```python
from build123d import *

# Parameters (mm, degrees)
SKETCH_1_R      = 2.1
EXTRUDE_1_DEPTH = 3


with BuildPart() as part:
    # 스케치1 → 보스-돌출1 (new, symmetric)
    with BuildSketch(Plane.XY):
        with BuildLine():
            Line((-4.654662174, -7.079831659), (-4.654662174, 5.301751688))
            Line((-4.654662174, 5.301751688), (10.655145319, 5.301751688))
            ThreePointArc((10.655145319, 5.301751688), (12.164725545, 4.600439307), (13.28874021, 3.372733093))
            Line((13.28874021, 3.372733093), (13.28874021, 2.168909846))
            ThreePointArc((13.28874021, 2.168909846), (11.333538367, 0.764001831), (8.927874518, 0.66724324))
            Line((8.927874518, 0.66724324), (3.345337826, 0.66724324))
            Line((3.345337826, 0.66724324), (3.345337826, -6.968753808))
            ThreePointArc((3.345337826, -6.968753808), (0.343177667, -8.564508011), (-0.439769501, -11.873041045))
            ThreePointArc((-0.439769501, -11.873041045), (-1.484211123, -14.014409685), (-3.830025316, -13.597907913))
            ThreePointArc((-3.830025316, -13.597907913), (-5.564151963, -10.506098848), (-4.654662174, -7.079831659))
        make_face()
        Circle(SKETCH_1_R, mode=Mode.SUBTRACT)
    extrude(amount=EXTRUDE_1_DEPTH, both=True)


solid = part.part
```
CAD build for the part. Positions are in the model's coordinates, mm. A direction names the side the tool comes from. Round coordinates to 2 decimals unless told otherwise and drop trailing zeros. Loops run counter-clockwise (first coordinate to the right, second up) from the corner with the lowest first, then second, coordinate; pieces in that order, holes last. Notation, with made-up numbers: M 9,21.5 L 36,21.5 A25 ccw 36,47.5 Z; hole C 33.5,26 d4. An arc over 180 degrees is marked long. Return JSON: item names as keys, results as strings. Group by question number.
(1) Tool access for faces 1 (the flat face through (3, 5.302, 0)), 2 (the flat face through (-4.655, -1, 0)), 3 (the flat face through (6, 0.667, 0)): list every direction of +Z, -Z, +X, -X, +Y, -Y with a clear straight run to the whole face (end or side of a thin tool).
(2) Saw through at C-C, the plane z = 0. List the corners of the cut face in (x, y), and give its area (3 significant figures).
(3) Saw through at B-B, the plane y = 0. List the corners of the cut face in (x, z).
(4) Saw through at A-A, the plane x = 0. List the corners of the cut face in (y, z).
(5) Mould opens along Y. For faces 4 (the cylindrical face through (12.15, 4.61, 0.04)), 5 (the cylindrical face through (0.37, -8.53, 0.04)), 6 (the flat face through (13.289, 3, 0)) say: +Y half, -Y half, draft (parallel to the pull), parting line (faces both ways), or undercut.
(6) Saw through at D-D, the plane y = 2.75. List the corners of the cut face in (x, z), and give its area (3 significant figures).
(7) Drop flat-ended pins along their axis: P1, Ø3, axis at x = 3.5, z = -1.5, coming from the -Y side; P2, Ø1.5, axis at x = 5.5, z = -1.5, coming from the -Y side; P3, Ø3, axis at y = 0, z = 1.5, coming from the +X side. Give the stop position or say it passes through.
(8) Wall check: probe 1 along Y at (x, z) = (4.75, -1.05); probe 2 along Y at (x, z) = (0, 1.55); probe 3 along X at (y, z) = (-1.5, 0.5). Give the ranges that are in metal, low to high. Write a range as [from, to].
Answer list:
{
 "1": {"face 1": "+Z, -Z, +X, -X, +Y", "face 2": "+Z, -Z, -X, +Y", "face 3": "+Z, -Z, -Y"},
 "2": {"outline": "M -4.65,-7.08 A4.72 ccw -3.83,-13.6 A1.98 ccw -0.44,-11.87 A4.12 cw 3.35,-6.97 L 3.35,0.67 L 8.93,0.67 A4.19 ccw 13.29,2.17 L 13.29,3.37 A4.25 ccw 10.66,5.3 L -4.65,5.3 Z; hole C 0,0 d4.2", "area": "163 mm2"},
 "3": {"outline": "M -4.65,-3 L -2.1,-3 L -2.1,3 L -4.65,3 Z; M 2.1,-3 L 3.35,-3 L 3.35,3 L 2.1,3 Z"},
 "4": {"outline": "M -9.09,-3 L -2.1,-3 L -2.1,3 L -9.09,3 Z; M 2.1,-3 L 5.3,-3 L 5.3,3 L 2.1,3 Z"},
 "5": {"face 4": "+Y half", "face 5": "undercut", "face 6": "draft"},
 "6": {"outline": "M -4.65,-3 L 13.29,-3 L 13.29,3 L -4.65,3 Z", "area": "108 mm2"},
 "7": {"P1": "y = -7.29", "P2": "y = 0.67", "P3": "x = 12.64"},
 "8": {"probe 1": "[0.67, 5.3]", "probe 2": "[-9.09, -2.1], [2.1, 5.3]", "probe 3": "[-4.65, -1.47], [1.47, 3.35]"}
}
